from build123d import *

# Parameters (mm, degrees)
EXTRUDE_1_DEPTH     = 8
FILLET_1_R          = 3
FILLET_2_R          = 5
SKETCH_2_R          = 14
CUT_EXTRUDE_1_DEPTH = 10
SKETCH_3_R          = 2.75
CUT_EXTRUDE_2_DEPTH = 10
SKETCH_4_R          = 11.5
SKETCH_4_R_2        = 2
CUT_EXTRUDE_3_DEPTH = 10


with BuildPart() as part:
    # 草图1 → 凸台-拉伸1 (new body)
    with BuildSketch(Plane.XY):
        Polygon((0, 0), (103, 0), (169.65, -5), (429.65, -5), (496.3, 0), (599.3, 0), (599.3, -60), (496.3, -60), (429.65, -55), (169.65, -55), (103, -60), (0, -60), align=None)
        Polygon((169.65, -30), (199.65, -20), (229.65, -30), (199.65, -40), align=None, mode=Mode.SUBTRACT)
        Polygon((269.65, -30), (299.65, -20), (329.65, -30), (299.65, -40), align=None, mode=Mode.SUBTRACT)
        Polygon((369.65, -30), (399.65, -20), (429.65, -30), (399.65, -40), align=None, mode=Mode.SUBTRACT)
    extrude(amount=EXTRUDE_1_DEPTH)

    # 圆角1
    fillet_1_edges = [part.edges().sort_by_distance(p)[0] for p in [
        (269.65, -30, 4),
        (299.65, -40, 4),
        (329.65, -30, 4),
        (299.65, -20, 4),
        (169.65, -30, 4),
        (199.65, -40, 4),
        (229.65, -30, 4),
        (199.65, -20, 4),
        (369.65, -30, 4),
        (399.65, -40, 4),
        (429.65, -30, 4),
        (399.65, -20, 4),
    ]]
    fillet(fillet_1_edges, radius=FILLET_1_R)

    # 圆角2
    fillet_2_edges = [part.edges().sort_by_distance(p)[0] for p in [
        (0, 0, 4),
        (599.3, 0, 4),
        (599.3, -60, 4),
        (0, -60, 4),
    ]]
    fillet(fillet_2_edges, radius=FILLET_2_R)

    # 草图2 → 切除-拉伸1 (cut)
    with BuildSketch(Plane.XY.offset(8)):
        with Locations((74.3, -30)):
            Circle(SKETCH_2_R)
        with Locations((525, -30)):
            Circle(SKETCH_2_R)
    extrude(amount=-CUT_EXTRUDE_1_DEPTH, mode=Mode.SUBTRACT)

    # 草图3 → 切除-拉伸2 (cut)
    with BuildSketch(Plane(origin=(0, 0, 0), x_dir=(-1, 0, 0), z_dir=(0, 0, -1))):
        with Locations((-537.05, -11)):
            Circle(SKETCH_3_R)
        with Locations((-513.05, -11)):
            Circle(SKETCH_3_R)
        with Locations((-513.05, -49)):
            Circle(SKETCH_3_R)
        with Locations((-537.05, -49)):
            Circle(SKETCH_3_R)
        with Locations(Location((-62.25, -49, 0), (0, 0, 180))):
            Circle(SKETCH_3_R)
        with Locations(Location((-86.25, -49, 0), (0, 0, 180))):
            Circle(SKETCH_3_R)
        with Locations(Location((-86.25, -11, 0), (0, 0, 180))):
            Circle(SKETCH_3_R)
        with Locations(Location((-62.25, -11, 0), (0, 0, 180))):
            Circle(SKETCH_3_R)
    extrude(amount=-CUT_EXTRUDE_2_DEPTH, mode=Mode.SUBTRACT)

    # 草图4 → 切除-拉伸3 (cut)
    with BuildSketch(Plane.XY.offset(8)):
        with Locations((20.8, -30)):
            Circle(SKETCH_4_R)
        with Locations((5.3, -14.5)):
            Circle(SKETCH_4_R_2)
        with Locations((36.3, -14.5)):
            Circle(SKETCH_4_R_2)
        with Locations((36.3, -45.5)):
            Circle(SKETCH_4_R_2)
        with Locations((5.3, -45.5)):
            Circle(SKETCH_4_R_2)
        with Locations((563, -45.5)):
            Circle(SKETCH_4_R_2)
        with Locations((594, -45.5)):
            Circle(SKETCH_4_R_2)
        with Locations((594, -14.5)):
            Circle(SKETCH_4_R_2)
        with Locations((563, -14.5)):
            Circle(SKETCH_4_R_2)
        with Locations((578.5, -30)):
            Circle(SKETCH_4_R)
    extrude(amount=-CUT_EXTRUDE_3_DEPTH, mode=Mode.SUBTRACT)


solid = part.part
Design review of the part built by this model. Coordinates are the model's own, in mm. Round coordinates to 2 decimals unless told otherwise and drop trailing zeros. Write each loop counter-clockwise with the first axis right and the second up, starting at its lowest first coordinate (ties: lowest second). Pieces come first, ordered by that corner, then holes. Notation, with made-up numbers: (83, -33) -> (110, -33) arc R25 cw to (110, -16) -> close; hole circle Ø10 at (70, 83.25). An arc over 180 degrees is marked (long way). One line per item, written item: value. Start each with the question number.
Q1. To check wall thickness, follow probe 1 along X at (y, z) = (-14, 6); probe 2 along Y at (x, z) = (5.3, 3); probe 3 along X at (y, z) = (-40, 5.75). State the ranges of each line that lie inside material, in increasing order.
Q2. Add section C-C (x = 360). Give the boundary of the cut face in (y, z).
Q3. The part is to be moulded in two halves that separate along Y. For faces 1 (the face through (589.123, -34.405, 4.056)), 2 (the face through (304, -43, 0)), say which applies: pulls with the +Y half, pulls with the -Y half, needs draft (parallel to the pull), parting line crosses it, or undercut.
Q4. Add section A-A (x = 74.3). Give the boundary of the cut face in (y, z).
Q5. Add section B-B (z = 1.75). State how many separate pieces and enclosed holes the cut face has, then the cut area to 3 significant figures.
Q6. Insertion check: P1, Ø9, axis at x = 513.05, y = -11, coming from the -Z side; P2, Ø4, axis at x = 294.5, z = 6, coming from the +Y side. Each pin has a flat end and moves straight along its axis. Give the tip position at first contact, or say it passes through.
Response:
1. probe 1: x = 0 to 3.36, 7.24 to 34.36, 38.24 to 561.06, 564.94 to 592.06, 595.94 to 599.3
1. probe 2: y = -60 to -47.5, -43.5 to -16.5, -12.5 to 0
1. probe 3: x = 0 to 15.12, 26.48 to 64.5, 84.1 to 515.2, 534.8 to 572.82, 584.18 to 599.3
2. outline: (-55, 0) -> (-5, 0) -> (-5, 8) -> (-55, 8) -> close
3. face 1: undercut
3. face 2: needs draft
4. outline: (-60, 0) -> (-44, 0) -> (-44, 8) -> (-60, 8) -> close; (-16, 0) -> (0, 0) -> (0, 8) -> (-16, 8) -> close
5. separate pieces: 1
5. enclosed holes: 23
5. area: 28,600 mm^2
6. P1: stops at z = 0
6. P2: stops at y = -5
